Input: part model. Units: mm. Frame: model coordinates. A direction names the side the tool comes from. Give positions to 0.01 mm unless a question says otherwise; leave off trailing zeros. Loops run counter-clockwise (first coordinate to the right, second up) from the corner with the lowest first, then second, coordinate; pieces in that order, holes last. Notation, with made-up numbers: (-9, -27) -> (3, -27) arc R12 ccw to (3, -21) -> close; hole circle Ø1 at (-2.75, -16). An arc over 180 degrees is marked (long way). Answer as a JSON object with one key per item and string values.
```python
from build123d import *

# Parameters (mm, degrees)
F0_R           = 12.7
F1_DEPTH       = 6.35
F3_DEPTH       = 3.175
F4_R           = 5.55625
F5_DEPTH       = 3.175
F6_R           = 3.96875
F7_DEPTH       = 8.73125
F8_R           = 2.2479
F9_DEPTH       = 15.08125
F11_DEPTH      = 6.35
F12_COUNT      = 12
F12_ANGLE      = 330
F14_END_RADIUS = 5.55625
F14_REACH      = 18.1506366107
F17_END_RADIUS = 5.55625
F17_REACH      = 35.6755158286


with BuildPart() as f1:
    # F0 (on Top) → F1 (new body)
    with BuildSketch(Plane.XY):
        Circle(F0_R)
    extrude(amount=F1_DEPTH)

    # F2 (on face) → F3 (cut)
    with BuildSketch(Plane(origin=(0, 0, 0), x_dir=(1, 0, 0), z_dir=(0, 0, -1))):
        Polygon((2.2913588808, 3.96875), (-2.2913588808, 3.96875), (-4.5827177617, 0), (-2.2913588808, -3.96875), (2.2913588808, -3.96875), (4.5827177617, 0), align=None)
    extrude(amount=-F3_DEPTH, mode=Mode.SUBTRACT)

    # F4 (on face) → F5 (join)
    with BuildSketch(Plane.XY.offset(6.35)):
        Circle(F4_R)
    extrude(amount=F5_DEPTH)

    # F6 (on face) → F7 (join)
    with BuildSketch(Plane.XY.offset(9.525)):
        Circle(F6_R)
    extrude(amount=F7_DEPTH)

    # F8 (on face) → F9 (cut, through all)
    with BuildSketch(Plane(origin=(0, 0, 3.175), x_dir=(1, 0, 0), z_dir=(0, 0, -1))):
        Circle(F8_R)
    extrude(amount=-F9_DEPTH, mode=Mode.SUBTRACT)

    # F10 (on face) → F11 (join, through all)
    with BuildSketch(Plane(origin=(0, 0, 0), x_dir=(1, 0, 0), z_dir=(0, 0, -1))):
        with BuildLine():
            ThreePointArc((-1.5843963802, 12.60078125), (0, 12.7), (1.5843963802, 12.60078125))
            ThreePointArc((1.5843963802, 12.60078125), (0, 14.2875), (-1.5843963802, 12.60078125))
        make_face()
    f11 = extrude(amount=-F11_DEPTH)

    # F12: F11 ×12 about axis
    f12_axis = Axis((0, 0, 0), (0, 0, -1))
    for i in range(1, F12_COUNT):
        add(f11.rotate(f12_axis, i * F12_ANGLE / (F12_COUNT - 1)))

    f14_end = (Plane(origin=(0, 0, 7.9375), x_dir=(-1, 0, 0), z_dir=(0, 0, -1)) * Cylinder(F14_END_RADIUS, 124.9884067655, mode=Mode.PRIVATE)).faces().sort_by_distance((-5.55625, 0, 7.9375))[0]
    # F13 (on Front) → F14 (cut, up to the whole of a round face its end follows)
    with BuildSketch(Plane.XZ):
        with BuildLine():
            ThreePointArc((0, 8.0772), (-1.7272, 6.35), (0, 4.6228))
            Line((0, 4.6228), (0, 8.0772))
        make_face()
        with BuildLine():
            Line((0, 8.0772), (0, 4.6228))
            ThreePointArc((0, 4.6228), (1.2213148325, 5.1286851675), (1.7272, 6.35))
            ThreePointArc((1.7272, 6.35), (1.2213148325, 7.5713148325), (0, 8.0772))
        make_face()
    f14_long = extrude(amount=F14_REACH, mode=Mode.PRIVATE)
    add(split(f14_long, bisect_by=f14_end, keep=Keep.BOTTOM, mode=Mode.PRIVATE), mode=Mode.SUBTRACT)

    f17_end = (Plane(origin=(0, 0, 7.9375), x_dir=(-1, 0, 0), z_dir=(0, 0, -1)) * Cylinder(F17_END_RADIUS, 160.0381652835, mode=Mode.PRIVATE)).faces().sort_by_distance((-5.55625, 0, 7.9375))[0]
    # F16 (on offset) → F17 (cut, up to the whole of a round face its end follows)
    with BuildSketch(Plane.XZ.offset(14.2875)):
        with BuildLine():
            Line((3.175, 6.35), (-3.175, 6.35))
            ThreePointArc((-3.175, 6.35), (0, 3.175), (3.175, 6.35))
        make_face()
    f17_long = extrude(amount=-F17_REACH, mode=Mode.PRIVATE)
    add(split(f17_long, bisect_by=f17_end, keep=Keep.ALL, mode=Mode.PRIVATE).solids().sort_by_distance((0, -14.2875, 5.0024881485))[0], mode=Mode.SUBTRACT)


solid = f1.part
```
Q1. Section C-C, the plane y = 4.5. Return the cut outline in (x, z) (3 decimals), then the cut area to 3 significant figures.
Evaluation:
{"outline": "(-11.876, 0) -> (11.876, 0) -> (11.876, 6.35) -> (3.259, 6.35) -> (3.259, 9.525) -> (-3.259, 9.525) -> (-3.259, 6.35) -> (-11.876, 6.35) -> close", "area": "172 mm2"}
Q2. Section D-D, the plane x = 6.35. Return the cut outline in (y, z), then the cut area to 3 significant figures.
Evaluation:
{"outline": "(-12.59, 0) -> (12.59, 0) -> (12.59, 6.35) -> (-12.59, 6.35) -> close", "area": "160 mm2"}
Q3. Draft query along X for faces 1 (the cylindrical face through (-12.274, -3.264, 3.131)), 2 (the flat face through (-3.42, -2.01, 1.57)), 3 (the flat face through (6, 1, 6.35)). Return one class per face: +X half, -X half, draft (parallel to the pull), parting line (faces both ways), or undercut.
Evaluation:
{"face 1": "-X half", "face 2": "undercut", "face 3": "draft"}
Q4. Access query for faces 4 (the cylindrical face through (-3.31, -12.26, 2.42)), 5 (the cylindrical face through (-12.26, 3.31, 3.13)), 6 (the flat face through (-4, 1, 9.525)). Directions: +Z, -Z, +X, -X, +Y, -Y. A direction counts if a zero-diameter tool reaches every point of the face in a straight line with its end or side. Return the directions, or none.
Evaluation:
{"face 4": "+Z, -Z, -Y", "face 5": "+Z, -Z, -X", "face 6": "+Z"}
Q5. Section B-B, the plane z = 10.75. Return the cut outline in (x, y).
Evaluation:
{"outline": "circle Ø7.94 at (0, 0); hole circle Ø4.5 at (0, 0)"}
Q6. Pin query (flat end, axial travel): pin 1 (8 mm diameter, centred on y = 9.5, z = 6.5, fed in from +X); pin 2 (10 mm diameter, centred on x = -11, y = 3, fed in from +Z); pin 3 (2.5 mm diameter, centred on x = 1.5, y = 0, fed in from -Z) (3 decimals). Return the tip coordinate at first contact, or that it passes through.
Evaluation:
{"pin 1": "stops at x = 12.59", "pin 2": "stops at z = 6.35", "pin 3": "stops at z = 3.175"}
Q7. Section A-A, the plane x = -0.5. Return the cut outline in (y, z) (3 decimals), then the cut area to 3 significant figures.
Evaluation:
{"outline": "(-14.207, 0) -> (-3.969, 0) -> (-3.969, 3.175) -> (-2.192, 3.175) -> (-2.192, 4.697) -> (-5.534, 4.697) -> (-5.534, 3.215) -> (-14.207, 3.215) -> close; (-5.534, 8.003) -> (-2.192, 8.003) -> (-2.192, 18.256) -> (-3.937, 18.256) -> (-3.937, 9.525) -> (-5.534, 9.525) -> close; (2.192, 3.175) -> (3.969, 3.175) -> (3.969, 0) -> (14.207, 0) -> (14.207, 6.35) -> (5.534, 6.35) -> (5.534, 9.525) -> (3.937, 9.525) -> (3.937, 18.256) -> (2.192, 18.256) -> close", "area": "155 mm2"}
Q8. Ray query, line 1 along X through (y, z) = (-7.75, 3); line 2 along Y through (x, z) = (0, 9.25). Return the intervals inside material, ascending.
Evaluation:
{"line 1": "x = -11.75 to -10.25, -10.06 to 10.06, 10.25 to 11.75", "line 2": "y = -5.56 to -2.25, 2.25 to 5.56"}
